Part print with two shaded views. Sizes in mm from the minimum x, y, z corner. A direction names the side the tool comes from. Round coordinates to 2 decimals unless told otherwise and drop trailing zeros. Write each loop counter-clockwise with the first axis right and the second up, starting at its lowest first coordinate (ties: lowest second). Pieces come first, ordered by that corner, then holes. Notation, with made-up numbers: (77.5, 68) -> (131.5, 68) arc R21 cw to (131.5, 103) -> close; hole circle Ø2 at (46.25, -4.75). An arc over 180 degrees is marked (long way). Return JSON: item names as keys, results as strings.
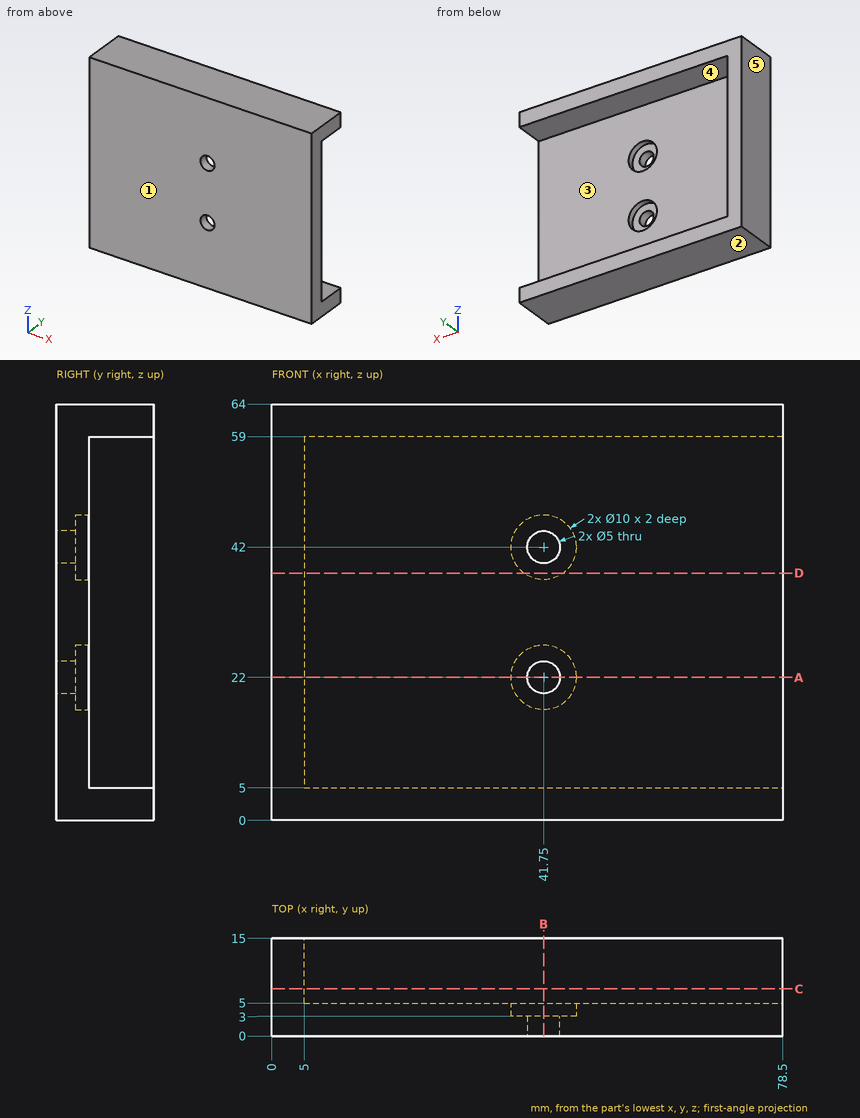
Q1. Wall check: L1, parallel to Z at x = 41.75, y = 2.25; L2, parallel to Z at x = 42, y = 3.75; L3, parallel to X at y = 4.3, z = 42. Give the ranges that are in metal, low to high.
Verdict:
{"L1": "z = 0 to 19.5, 24.5 to 39.5, 44.5 to 64", "L2": "z = 0 to 17.01, 26.99 to 37.01, 46.99 to 64", "L3": "x = 0 to 36.75, 46.75 to 78.5"}
Q2. Two-plate mould, pull along Z, no slides. Class the marked faces 1, 2 and 3: +Z half, -Z half, draft (parallel to the pull), parting line (faces both ways), or undercut.
Verdict:
{"face 1": "draft", "face 2": "-Z half", "face 3": "undercut"}
Q3. Saw through at B-B on x = 41.75. List the corners of the cut face in (y, z).
Verdict:
{"outline": "(0, 0) -> (15, 0) -> (15, 5) -> (5, 5) -> (5, 17) -> (3, 17) -> (3, 19.5) -> (0, 19.5) -> close; (0, 24.5) -> (3, 24.5) -> (3, 27) -> (5, 27) -> (5, 37) -> (3, 37) -> (3, 39.5) -> (0, 39.5) -> close; (0, 44.5) -> (3, 44.5) -> (3, 47) -> (5, 47) -> (5, 59) -> (15, 59) -> (15, 64) -> (0, 64) -> close"}
Q4. Pin check, flat tips, straight feed: pin 1 Ø4 at (x, z) = (10, 27.5) entering from +Y; pin 2 Ø6 at (x, z) = (41.75, 42) entering from +Y. Stop position of each tip, or through.
Verdict:
{"pin 1": "stops at y = 5", "pin 2": "stops at y = 3"}
Q5. 3-axis set-ups, long thin cutter, end or side, ignore diameter. For the marked faces 4 and 5: which of +Z, -Z, +X, -X, +Y, -Y reach the whole face in a straight line?
Verdict:
{"face 4": "+X, +Y", "face 5": "+Z, -Z, -X, +Y, -Y"}
Q6. Saw through at C-C on y = 7.25. List the corners of the cut face in (x, z).
Verdict:
{"outline": "(0, 0) -> (78.5, 0) -> (78.5, 5) -> (5, 5) -> (5, 59) -> (78.5, 59) -> (78.5, 64) -> (0, 64) -> close"}
Q7. Saw through at A-A on z = 22. List the corners of the cut face in (x, y), then the cut area to 4 significant figures.
Verdict:
{"outline": "(0, 0) -> (39.25, 0) -> (39.25, 3) -> (36.75, 3) -> (36.75, 5) -> (5, 5) -> (5, 15) -> (0, 15) -> close; (44.25, 0) -> (78.5, 0) -> (78.5, 5) -> (46.75, 5) -> (46.75, 3) -> (44.25, 3) -> close", "area": "407.5 mm²"}
Q8. Saw through at D-D on z = 38. List the corners of the cut face in (x, y), then the cut area to 4 significant figures.
Verdict:
{"outline": "(0, 0) -> (78.5, 0) -> (78.5, 5) -> (44.75, 5) -> (44.75, 3) -> (38.75, 3) -> (38.75, 5) -> (5, 5) -> (5, 15) -> (0, 15) -> close", "area": "430.5 mm²"}
